```python
from build123d import *

# Parameters (mm, degrees)
SKETCH1_R                              = 5
SKETCH1_R_2                            = 3
BOSS_EXTRUDE1_DEPTH                    = 2
SKETCH1_3_R                            = 5
SKETCH1_3_R_2                          = 3
BOSS_EXTRUDE2_DEPTH                    = 5
CHAMFER1_SIZE                          = 0.25
SKETCH5_R                              = 6.35
BOSS_EXTRUDE4_DEPTH                    = 12.5
F_3_8_0_375_DIAMETER_HOLE1_D           = 9.525
F_3_8_0_375_DIAMETER_HOLE1_DEPTH       = 12.08333524
F_3_8_0_375_DIAMETER_HOLE1_CSINK_D     = 10.795
F_3_8_0_375_DIAMETER_HOLE1_CSINK_ANGLE = 90
F_3_8_0_375_DIAMETER_HOLE1_TIP         = 0.41666476
CHAMFER2_SIZE                          = 0.25
CHAMFER3_SIZE                          = 0.5


with BuildPart() as part:
    # Sketch1 → Boss-Extrude1 (new body)
    with BuildSketch(Plane(origin=(0, 0, 0), x_dir=(1, 0, 0), z_dir=(0, 1, 0))):
        with Locations(Location((0, 0, 0), (0, 0, 270))):
            Circle(SKETCH1_R)
        Circle(SKETCH1_R_2, mode=Mode.SUBTRACT)
        Circle(SKETCH1_R_2)
    extrude(amount=BOSS_EXTRUDE1_DEPTH)

    # Sketch1_3 → Boss-Extrude2 (add)
    with BuildSketch(Plane(origin=(0, 0, 0), x_dir=(1, 0, 0), z_dir=(0, 1, 0))):
        with Locations(Location((0, 0, 0), (0, 0, 270))):
            Circle(SKETCH1_3_R)
        with Locations(Location((0, 0, 0), (0, 0, 270))):
            Circle(SKETCH1_3_R_2, mode=Mode.SUBTRACT)
    extrude(amount=BOSS_EXTRUDE2_DEPTH)

    # Chamfer1
    chamfer1_edges = [part.edges().sort_by_distance(p)[0] for p in [
        (0, 2, -3),
        (0, 5, -5),
        (0, 5, -3),
    ]]
    chamfer(chamfer1_edges, length=CHAMFER1_SIZE)

    # Sketch5 → Boss-Extrude4 (add)
    with BuildSketch(Plane(origin=(0, 0, 0), x_dir=(1, 0, 0), z_dir=(0, 1, 0))):
        with Locations(Location((0, 0, 0), (0, 0, 270))):
            Circle(SKETCH5_R)
    extrude(amount=-BOSS_EXTRUDE4_DEPTH)

    # 3_8 _0.375_ Diameter Hole1
    with Locations(Plane(origin=(0, -12.5, 0), x_dir=(-1, 0, 0), z_dir=(0, -1, 0))):
        with Locations((0, 0)):
            CounterSinkHole(F_3_8_0_375_DIAMETER_HOLE1_D / 2, F_3_8_0_375_DIAMETER_HOLE1_CSINK_D / 2, depth=F_3_8_0_375_DIAMETER_HOLE1_DEPTH, counter_sink_angle=F_3_8_0_375_DIAMETER_HOLE1_CSINK_ANGLE)
            with Locations((0, 0, -(F_3_8_0_375_DIAMETER_HOLE1_DEPTH + F_3_8_0_375_DIAMETER_HOLE1_TIP / 2))):  # 170° drill point
                Cone(0, F_3_8_0_375_DIAMETER_HOLE1_D / 2, F_3_8_0_375_DIAMETER_HOLE1_TIP, mode=Mode.SUBTRACT)

    # Chamfer2
    chamfer2_edges = [part.edges().sort_by_distance(p)[0] for p in [
        (0, -12.5, -6.35),
        (0, 0, -6.35),
    ]]
    chamfer(chamfer2_edges, length=CHAMFER2_SIZE)

    # Chamfer3
    chamfer3_edges = [part.edges().sort_by_distance(p)[0] for p in [
        (0, 0, -5),
    ]]
    chamfer(chamfer3_edges, length=CHAMFER3_SIZE)


solid = part.part
```
Work out the finished part from the listing and answer in its coordinate system (mm). A direction names the side the tool comes from. Give positions to 0.01 mm unless a question says otherwise; leave off trailing zeros. Write each loop counter-clockwise with the first axis right and the second up, starting at its lowest first coordinate (ties: lowest second). Pieces come first, ordered by that corner, then holes. Notation, with made-up numbers: (85.5, 70.25) -> (99.5, 70.25) arc R22 ccw to (99.5, 109.25) -> close; hole circle Ø11 at (60.25, 88.25). An arc over 180 degrees is marked (long way). Write item = value, one per line.
Q1. Section B-B on y = 1 is taken. Determine the outline of the cut face in (x, z), and give its area (3 significant figures).
Computed values:
outline = circle Ø10 at (0, 0)
area = 78.5 mm^2
Q2. Consider line 1 along Z through (x, y) = (4, 2.25); line 2 along Z through (x, y) = (2.25, -2.25); line 3 along Z through (x, y) = (-3, -11.5). Determine where each line is inside the solid, lowest interval first.
Computed values:
line_1 = -3 to 3
line_2 = -5.94 to -4.2, 4.2 to 5.94
line_3 = -5.6 to -3.7, 3.7 to 5.6
Q3. A tool of negligible diameter and unlimited length cuts with its end or side. For faces 1 (the flat face through (0, 2, 0)), 2 (the cylindrical face through (-3.78, -6.06, 2.9)), 3 (the cylindrical face through (-3.86, -6.17, -5.04)), from which of +Z, -Z, +X, -X, +Y, -Y can it reach the whole face along a straight path? Write none if from no direction.
Computed values:
face_1 = +Y
face_2 = -Y
face_3 = +Y, -Y
Q4. Section C-C on y = 3.5 is taken. Determine the outline of the cut face in (x, z).
Computed values:
outline = circle Ø10 at (0, 0); hole circle Ø6 at (0, 0)
Q5. A flat-ended cylindrical pin translates along its axis: pin 1 Ø4 at (x, z) = (-1, -2.5) entering from -Y. Find the tip coordinate at first contact, or state that the pin passes through.
Computed values:
pin_1 = -0.41
